Design review of the part built by this model. Coordinates are the model's own, in mm. Face numbers are marked on the shaded views. A direction names the side the tool comes from. Give positions to 0.01 mm unless a question says otherwise; leave off trailing zeros. Loops run counter-clockwise (first coordinate to the right, second up) from the corner with the lowest first, then second, coordinate; pieces in that order, holes last. Notation, with made-up numbers: (64.25, 38) -> (78.25, 38) arc R16 cw to (78.25, 65) -> close; hole circle Ø1 at (37.25, -8). An arc over 180 degrees is marked (long way). Answer in a Markdown table with one row per item. Add a question column.
(1) For pin 1 (7.5 mm diameter, centred on x = 678, y = 106.5, fed in from -Z); pin 2 (7.5 mm diameter, centred on x = 676.5, z = 103.5, fed in from -Y); pin 3 (1 mm diameter, centred on y = 49, z = 31, fed in from -X), all flat-tipped, find the tip position at first contact; note any pin that passes through.
(2) Consider section C-C on y = 26. Write out the cut boundary in (x, z).
(3) Consider section B-B on x = 0. Write out the cut boundary in (y, z).
(4) Draft analysis for pull direction X (two halves, no side actions). For the marked faces 1, 2 and 3, state which applies: +X half, -X half, draft (parallel to the pull), parting line (faces both ways), or undercut.
(5) For line 1 (Z direction, x = 0, y = 42); line 2 (X direction, y = 48, z = 63); line 3 (X direction, y = 37, z = 128.5), list the stretches that pass through material, from the lowest coordinate up.
(6) Consider section D-D on x = 237.5. Write out the cut boundary in (y, z), then the cut area to 3 significant figures.
(7) Consider section A-A on z = 63.5. Write out the cut boundary in (x, y), then the cut area to 3 significant figures.
(8) For the marked faces 4 and 5, list the 3-axis set-ups (+Z, -Z, +X, -X, +Y, -Y) from which the entire face can be reached by the end or side of a thin tool; tool diameter is ignored.
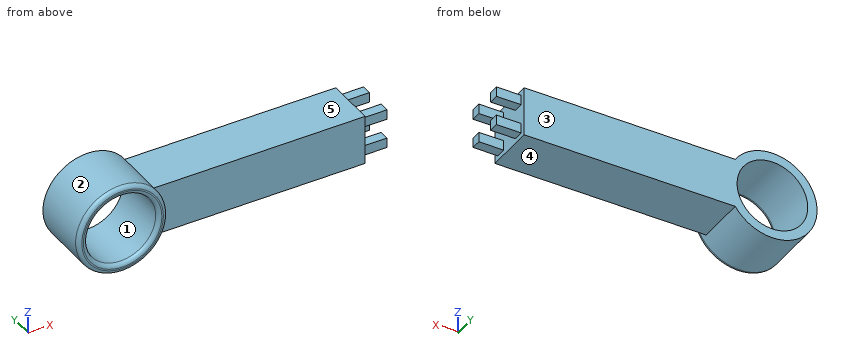
from build123d import *

# Parameters (mm, degrees)
SKETCH2_W               = 635
SKETCH2_H               = 127
BOSS_EXTRUDE1_DEPTH     = 127
SKETCH3_R               = 114.3
SKETCH3_R_2             = 90.424
BOSS_EXTRUDE2_DEPTH     = 152.4
SKETCH4_R               = 90.424
CUT_EXTRUDE2_DEPTH      = 1
CUT_EXTRUDE2_DEPTH_BACK = 153.4
SKETCH5_W               = 25.4
SKETCH5_H               = 25.4
BOSS_EXTRUDE3_DEPTH     = 63.5
FILLET1_R               = 10


with BuildPart() as part:
    # Sketch2 → Boss-Extrude1 (new body)
    with BuildSketch(Plane.XY):
        with Locations((317.5, 63.5)):
            Rectangle(SKETCH2_W, SKETCH2_H)
    extrude(amount=BOSS_EXTRUDE1_DEPTH)

    # Sketch3 → Boss-Extrude2 (add)
    with BuildSketch(Plane(origin=(0, 127, 0), x_dir=(1, 0, 0), z_dir=(0, 1, 0))):
        with Locations((0, -63.5)):
            Circle(SKETCH3_R)
        with Locations((0, -63.5)):
            Circle(SKETCH3_R_2, mode=Mode.SUBTRACT)
    extrude(amount=-BOSS_EXTRUDE2_DEPTH)

    # Sketch4 → Cut-Extrude2 (cut, two sides)
    with BuildSketch(Plane(origin=(0, 127, 0), x_dir=(1, 0, 0), z_dir=(0, 1, 0))) as cut_extrude2_sk:
        with Locations((0, -63.5)):
            Circle(SKETCH4_R)
    extrude(amount=CUT_EXTRUDE2_DEPTH, mode=Mode.SUBTRACT)
    extrude(cut_extrude2_sk.sketch, amount=-CUT_EXTRUDE2_DEPTH_BACK, mode=Mode.SUBTRACT)

    # Sketch5 → Boss-Extrude3 (add)
    with BuildSketch(Plane(origin=(635, 0, 0), x_dir=(0, 0, -1), z_dir=(1, 0, 0))):
        with Locations((-101.6, 101.6)):
            Rectangle(SKETCH5_W, SKETCH5_H)
        with Locations((-25.4, 25.4)):
            Rectangle(SKETCH5_W, SKETCH5_H)
        with Locations((-101.6, 25.4)):
            Rectangle(SKETCH5_W, SKETCH5_H)
        with Locations((-25.4, 101.6)):
            Rectangle(SKETCH5_W, SKETCH5_H)
    extrude(amount=BOSS_EXTRUDE3_DEPTH)

    # Fillet1
    fillet1_edges = [part.edges().sort_by_distance(p)[0] for p in [
        (-114.3, -25.4, 63.5),
        (-90.424, -25.4, 63.5),
    ]]
    fillet(fillet1_edges, radius=FILLET1_R)


solid = part.part
Values follow:
| question | item | result |
|---|---|---|
| 1 | pin 1 | z = 12.7 |
| 1 | pin 2 | y = 12.7 |
| 1 | pin 3 | x = -109.73 |
| 2 | outline | (95.04, 0) -> (635, 0) -> (635, 12.7) -> (698.5, 12.7) -> (698.5, 38.1) -> (635, 38.1) -> (635, 88.9) -> (698.5, 88.9) -> (698.5, 114.3) -> (635, 114.3) -> (635, 127) -> (95.04, 127) arc R114.3 ccw (long way) to start; hole circle Ø180.85 at (0, 63.5) |
| 3 | outline | (-25.4, -40.8) arc R10 ccw to (-15.4, -50.8) -> (127, -50.8) -> (127, -26.92) -> (-15.4, -26.92) arc R10 ccw to (-25.4, -36.92) -> close; (-25.4, 163.92) arc R10 ccw to (-15.4, 153.92) -> (127, 153.92) -> (127, 177.8) -> (-15.4, 177.8) arc R10 ccw to (-25.4, 167.8) -> close |
| 4 | face 1 | undercut |
| 4 | face 2 | parting line |
| 4 | face 3 | draft |
| 5 | line 1 | -50.8 to -26.92, 153.92 to 177.8 |
| 5 | line 2 | -114.3 to -90.42, 90.42 to 635 |
| 5 | line 3 | -94.02 to -62.86, 62.86 to 94.02 |
| 6 | outline | (0, 0) -> (127, 0) -> (127, 127) -> (0, 127) -> close |
| 6 | area | 16,100 mm2 |
| 7 | outline | (-114.3, -15.4) arc R10 ccw to (-104.3, -25.4) -> (-100.42, -25.4) arc R10 ccw to (-90.42, -15.4) -> (-90.42, 127) -> (-114.3, 127) -> close; (90.42, -15.4) arc R10 ccw to (100.42, -25.4) -> (104.3, -25.4) arc R10 ccw to (114.3, -15.4) -> (114.3, 0) -> (635, 0) -> (635, 127) -> (90.42, 127) -> close |
| 7 | area | 73,300 mm2 |
| 8 | face 4 | -Z, +X, +Y, -Y |
| 8 | face 5 | +Z, +X, +Y, -Y |
